from build123d import *

# Parameters (mm, degrees)
F0_R     = 11
F1_DEPTH = 6.96
F2_DEPTH = 6.96


with BuildPart() as f1:
    # F0 (on Front) → F1 (new body)
    with BuildSketch(Plane.XZ):
        Circle(F0_R)
        with BuildLine():
            ThreePointArc((-0.086483, 0.004757), (-0.057789, 0.064517), (0.004757, 0.086483))
            Line((0.004757, 0.086483), (0.002379, 0.043242))
            ThreePointArc((0.002379, 0.043242), (0.031452, 0.02977), (0.043307, 0))
            ThreePointArc((0.043307, 0), (0.043291, -0.00119), (0.043242, -0.002379))
            ThreePointArc((0.043242, -0.002379), (0.028895, -0.032258), (-0.002379, -0.043242))
            ThreePointArc((-0.002379, -0.043242), (-0.032258, -0.028895), (-0.043242, 0.002379))
            Line((-0.043242, 0.002379), (-0.086483, 0.004757))
        make_face(mode=Mode.SUBTRACT)
        Polygon((11.922232, 11.811606), (2.092604, 38.042489), (-10.284935, 13.26174), (-38.042489, 2.092604), (-11.041482, -12.638802), (-2.092604, -38.042489), (11.922232, -13.172698), (38.042489, -2.092604), align=None)
        Circle(F0_R, mode=Mode.SUBTRACT)
    extrude(amount=F1_DEPTH)

    # F0 (on Front) → F2 (join)
    with BuildSketch(Plane.XZ):
        Circle(F0_R)
        with BuildLine():
            ThreePointArc((-0.086483, 0.004757), (-0.057789, 0.064517), (0.004757, 0.086483))
            Line((0.004757, 0.086483), (0.002379, 0.043242))
            ThreePointArc((0.002379, 0.043242), (0.031452, 0.02977), (0.043307, 0))
            ThreePointArc((0.043307, 0), (0.043291, -0.00119), (0.043242, -0.002379))
            ThreePointArc((0.043242, -0.002379), (0.028895, -0.032258), (-0.002379, -0.043242))
            ThreePointArc((-0.002379, -0.043242), (-0.032258, -0.028895), (-0.043242, 0.002379))
            Line((-0.043242, 0.002379), (-0.086483, 0.004757))
        make_face(mode=Mode.SUBTRACT)
        Polygon((11.922232, 11.811606), (2.092604, 38.042489), (-10.284935, 13.26174), (-38.042489, 2.092604), (-11.041482, -12.638802), (-2.092604, -38.042489), (11.922232, -13.172698), (38.042489, -2.092604), align=None)
        Circle(F0_R, mode=Mode.SUBTRACT)
    extrude(amount=F2_DEPTH)


solid = f1.part
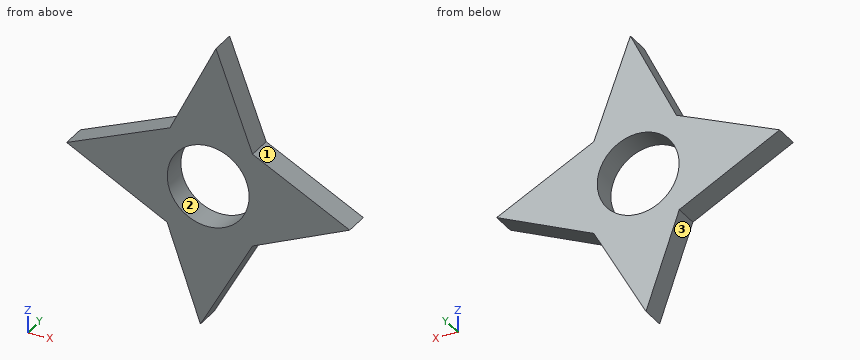
Build history of the part. All positions in model axes, mm. Face numbers are marked on the shaded views. Round coordinates to 2 decimals unless told otherwise and drop trailing zeros. Write each loop counter-clockwise with the first axis right and the second up, starting at its lowest first coordinate (ties: lowest second). Pieces come first, ordered by that corner, then holes. Notation, with made-up numbers: M 56,81.5 L 106,81.5 A24 cw 106,105.5 Z; hole C 28,61 d3. An arc over 180 degrees is marked long. Answer in a Markdown table with one row per item.
1. Probe L1, parallel to Z at x = 0, y = -5; L2, parallel to X at y = -0.5, z = -2.5; L3, parallel to X at y = -2.75, z = 9. List the from-to ranges inside material, lowest first. Write a range as [from, to].
Geometry check:
| item | result |
|---|---|
| L1 | [-34.33, -11], [11, 33.85] |
| L2 | [-29.62, -10.71], [10.71, 37.08] |
| L3 | [-20.88, -6.32], [6.32, 17.2] |
2. Saw through at D-D (z = 15.5). List the corners of the cut face in (x, y).
Geometry check:
| item | result |
|---|---|
| outline | M -9.17,-6.96 L 10.54,-6.96 L 10.54,0 L -9.17,0 Z |
3. Mould opens along X. For the marked faces 1, 2 and 3 say: +X half, -X half, draft (parallel to the pull), parting line (faces both ways), or undercut.
Geometry check:
| item | result |
|---|---|
| face 1 | +X half |
| face 2 | undercut |
| face 3 | -X half |
4. Saw through at B-B (x = 9). List the corners of the cut face in (y, z), and give its area (3 significant figures).
Geometry check:
| item | result |
|---|---|
| outline | M -6.96,-18.36 L 0,-18.36 L 0,-6.32 L -6.96,-6.32 Z; M -6.96,6.32 L 0,6.32 L 0,19.61 L -6.96,19.61 Z |
| area | 176 mm2 |
5. Saw through at C-C (z = -7). List the corners of the cut face in (x, y), and give its area (3 significant figures).
Geometry check:
| item | result |
|---|---|
| outline | M -21.38,-6.96 L -8.49,-6.96 L -8.49,0 L -21.38,0 Z; M 8.49,-6.96 L 26.47,-6.96 L 26.47,0 L 8.49,0 Z |
| area | 215 mm2 |
6. Saw through at A-A (y = -4). List the corners of the cut face in (x, z), and give its area (3 significant figures).
Geometry check:
| item | result |
|---|---|
| outline | M -38.04,2.09 L -11.04,-12.64 L -2.09,-38.04 L 11.92,-13.17 L 38.04,-2.09 L 11.92,11.81 L 2.09,38.04 L -10.28,13.26 Z; hole C 0,0 d22 |
| area | 1,450 mm2 |
7. Flat gauge pins, fed straight in: P1, Ø1.5, axis at x = 2, y = -5.5, coming from the -Z side; P2, Ø3, axis at x = 29, y = -3, coming from the -Z side; P3, Ø1, axis at x = -13, y = -5.5, coming from the -Z side. Where does each tip first touch, or does it go through?
Geometry check:
| item | result |
|---|---|
| P1 | z = -32.11 |
| P2 | z = -6.56 |
| P3 | z = -11.84 |
